Build history of the part. All positions in model axes, mm. Coordinates: 2 decimals unless noted, no trailing zeros. Write each loop counter-clockwise with the first axis right and the second up, starting at its lowest first coordinate (ties: lowest second). Pieces come first, ordered by that corner, then holes.
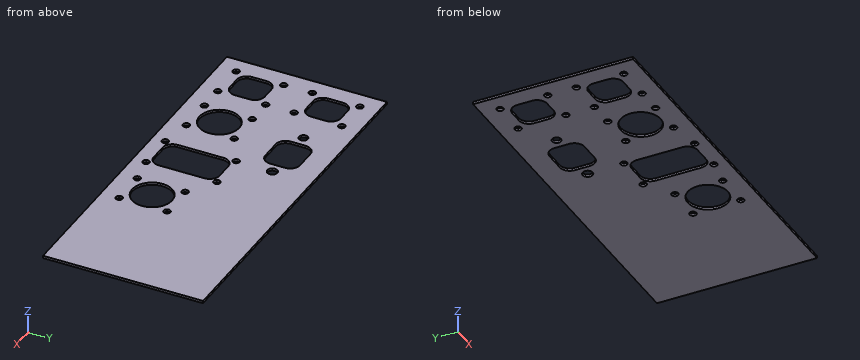
Autodesk Inventor part; units mm, degrees
ref_plane "YZ Plane" through (0, 0, 0) normal (1, 0, 0) x (0, 1, 0)
ref_plane "XZ Plane" through (0, 0, 0) normal (0, 1, 0) x (-1, 0, 0)
ref_plane "XY Plane" through (0, 0, 0) normal (0, 0, 1) x (1, 0, 0)
sketch "Sketch1" plane through (0, 0, 0) normal (0, 0, 1) x (1, 0, 0)
  line L0 (0, 0) -> (228.6, 0)
  line L1 (228.6, 0) -> (228.6, -101.6)
  line L2 (228.6, -101.6) -> (0, -101.6)
  line L3 (0, -101.6) -> (0, 0)
  dimension "d0" = 101.6
  dimension "d1" = 228.6
extrude "Extrusion1" add sketch "Sketch1" along normal blind 1.5875
sketch "Sketch2" plane through (0, 0, 1.5875) normal (0, 0, 1) x (1, 0, 0)
  line L0 (18.3388, -37.6555) -> (26.6192, -37.6555)
  line L1 (32.9692, -31.3055) -> (32.9692, -21.9075)
  line L2 (26.6192, -15.5575) -> (18.3388, -15.5575)
  line L3 (11.9888, -21.9075) -> (11.9888, -31.3055)
  arc A0 (11.9888, -31.3055) -> (18.3388, -37.6555) centre (18.3388, -31.3055) ccw
  arc A1 (18.3388, -15.5575) -> (11.9888, -21.9075) centre (18.3388, -21.9075) ccw
  arc A2 (32.9692, -21.9075) -> (26.6192, -15.5575) centre (26.6192, -21.9075) ccw
  arc A3 (26.6192, -37.6555) -> (32.9692, -31.3055) centre (26.6192, -31.3055) ccw
  circle A4 centre (10.9982, -41.783) radius 2.1463
  circle A5 centre (33.7058, -11.43) radius 2.1463
  circle A6 centre (33.7058, -41.783) radius 2.1463
  circle A7 centre (11.2522, -11.43) radius 2.1463
  line L4 (6.35, -46.863) -> (38.1, -46.863)
  line L5 (38.1, -46.863) -> (38.1, -6.35)
  line L6 (38.1, -6.35) -> (6.35, -6.35)
  line L7 (6.35, -6.35) -> (6.35, -46.863)
  line L8 (228.6, 0) -> (0, 0)
  line L9 (0, 0) -> (0, -101.6)
  point P0 (32.9692, -15.5575)
  point P1 (32.9692, -37.6555)
  point P2 (11.9888, -15.5575)
  dimension "d4" = 20.9804
  dimension "d5" = 22.098
  dimension "d6" = 6.35
  dimension "d7" = 4.2926
  dimension "d8" = 4.2926
  dimension "d9" = 4.2926
  dimension "d10" = 4.2926
  dimension "d11" = 0.9906
  dimension "d12" = 0.7366
  dimension "d13" = 0.7366
  dimension "d14" = 0.7366
  dimension "d15" = 4.1275
  dimension "d16" = 4.1275
  dimension "d17" = 4.1275
  dimension "d18" = 4.1275
  dimension "d19" = 31.75
  dimension "d20" = 40.513
  dimension "d21" = 5.08
  dimension "d22" = 4.6482
  dimension "d26" = 6.35
  dimension "d27" = 6.35
extrude "J9" cut sketch "Sketch2" against normal blind 1.5875 contours A0 L3 A1 L2 A2 L1 A3 L0 | A4 | A5 | A6 | A7
sketch "Sketch3" plane through (0, 0, 1.5875) normal (0, 0, 1) x (1, 0, 0)
  line L0 (67.183, -36.3982) -> (79.9084, -36.3982)
  line L1 (86.2584, -30.0482) -> (86.2584, -20.6502)
  line L2 (79.9084, -14.3002) -> (67.183, -14.3002)
  line L3 (60.833, -20.6502) -> (60.833, -30.0482)
  arc A0 (60.833, -30.0482) -> (67.183, -36.3982) centre (67.183, -30.0482) ccw
  arc A1 (79.9084, -36.3982) -> (86.2584, -30.0482) centre (79.9084, -30.0482) ccw
  arc A2 (86.2584, -20.6502) -> (79.9084, -14.3002) centre (79.9084, -20.6502) ccw
  arc A3 (67.183, -14.3002) -> (60.833, -20.6502) centre (67.183, -20.6502) ccw
  circle A4 centre (54.2417, -25.3492) radius 2.8067
  circle A5 centre (92.8497, -25.3492) radius 3.175
  line L4 (45.6692, -40.8432) -> (100.4062, -40.8432)
  line L5 (100.4062, -40.8432) -> (100.4062, -9.8552)
  line L6 (100.4062, -9.8552) -> (45.6692, -9.8552)
  line L7 (45.6692, -9.8552) -> (45.6692, -40.8432)
  line L8 (228.6, 0) -> (0, 0)
  line L9 (32.9692, -21.9075) -> (32.9692, -31.3055)
  dimension "d30" = 6.35
  dimension "d31" = 25.4254
  dimension "d32" = 22.098
  dimension "d33" = 5.6134
  dimension "d34" = 6.35
  dimension "d35" = 6.5913
  dimension "d36" = 6.5913
  dimension "d37" = 11.049
  dimension "d38" = 11.049
  dimension "d39" = 54.737
  dimension "d40" = 30.988
  dimension "d41" = 15.494
  dimension "d42" = 14.1478
  dimension "d98" = 12.7
  dimension "d99" = 9.8552
extrude "J8" cut sketch "Sketch3" against normal blind 1.5875 contours A0 L3 A3 L2 A2 L1 A1 L0 | A4 | A5
sketch "Sketch4" plane through (0, 0, 1.5875) normal (0, 0, 1) x (1, 0, 0)
  circle A0 centre (61.5442, -74.9935) radius 12.7
  circle A1 centre (50.3174, -90.17) radius 2.159
  circle A2 centre (50.3174, -59.817) radius 2.159
  circle A3 centre (72.771, -90.17) radius 2.159
  circle A4 centre (72.771, -59.817) radius 2.159
  line L0 (45.6692, -95.25) -> (77.4192, -95.25)
  line L1 (77.4192, -95.25) -> (77.4192, -54.737)
  line L2 (77.4192, -54.737) -> (45.6692, -54.737)
  line L3 (45.6692, -54.737) -> (45.6692, -95.25)
  line L4 (228.6, 0) -> (0, 0)
  line L5 (0, 0) -> (0, -101.6)
  line L6 (0, -101.6) -> (228.6, -101.6)
  line L7 (32.9692, -21.9075) -> (32.9692, -31.3055)
  dimension "d49" = 25.4
  dimension "d50" = 4.318
  dimension "d51" = 4.318
  dimension "d52" = 4.318
  dimension "d53" = 4.318
  dimension "d54" = 11.2268
  dimension "d55" = 11.2268
  dimension "d56" = 11.2268
  dimension "d57" = 11.2268
  dimension "d58" = 15.1765
  dimension "d59" = 15.1765
  dimension "d60" = 15.1765
  dimension "d61" = 15.1765
  dimension "d62" = 31.75
  dimension "d63" = 40.513
  dimension "d64" = 5.08
  dimension "d65" = 4.6482
  dimension "d69" = 6.35
  dimension "d97" = 12.7
extrude "J7" cut sketch "Sketch4" against normal blind 1.5875 contours A0 | A1 | A2 | A3 | A4
sketch "Sketch5" plane through (0, 0, 1.5875) normal (0, 0, 1) x (1, 0, 0)
  arc A0 (18.3388, -63.9445) -> (11.9888, -70.2945) centre (18.3388, -70.2945) ccw
  line L0 (32.9692, -79.6925) -> (32.9692, -70.2945)
  circle A1 centre (11.2522, -59.817) radius 2.1463
  line L1 (38.1, -54.737) -> (6.35, -54.737)
  line L2 (11.9888, -70.2945) -> (11.9888, -79.6925)
  line L3 (18.3388, -86.0425) -> (26.6192, -86.0425)
  line L4 (38.1, -95.25) -> (38.1, -54.737)
  line L5 (6.35, -54.737) -> (6.35, -95.25)
  line L6 (26.6192, -63.9445) -> (18.3388, -63.9445)
  circle A2 centre (33.7058, -59.817) radius 2.1463
  arc A3 (11.9888, -79.6925) -> (18.3388, -86.0425) centre (18.3388, -79.6925) ccw
  arc A4 (26.6192, -86.0425) -> (32.9692, -79.6925) centre (26.6192, -79.6925) ccw
  circle A5 centre (10.9982, -90.17) radius 2.1463
  circle A6 centre (33.7058, -90.17) radius 2.1463
  line L7 (6.35, -95.25) -> (38.1, -95.25)
  arc A7 (32.9692, -70.2945) -> (26.6192, -63.9445) centre (26.6192, -70.2945) ccw
  line L8 (228.6, 0) -> (0, 0)
  line L9 (0, 0) -> (0, -101.6)
  line L10 (0, -101.6) -> (228.6, -101.6)
  point P0 (11.9888, -63.9445)
  point P1 (32.9692, -63.9445)
  point P2 (32.9692, -86.0425)
  dimension "d72" = 20.9804
  dimension "d73" = 22.098
  dimension "d74" = 6.35
  dimension "d75" = 4.2926
  dimension "d76" = 4.2926
  dimension "d77" = 4.2926
  dimension "d78" = 4.2926
  dimension "d79" = 0.9906
  dimension "d80" = 0.7366
  dimension "d81" = 0.7366
  dimension "d82" = 0.7366
  dimension "d83" = 4.1275
  dimension "d84" = 4.1275
  dimension "d85" = 4.1275
  dimension "d86" = 4.1275
  dimension "d87" = 31.75
  dimension "d88" = 40.513
  dimension "d89" = 5.08
  dimension "d90" = 4.6482
  dimension "d93" = 6.35
  dimension "d94" = 6.35
extrude "J6" cut sketch "Sketch5" against normal blind 1.5875 contours L6 A7 L0 A4 L3 A3 L2 A0 | A1 | A2 | A5 | A6
sketch "Sketch6" plane through (0, 0, 1.5875) normal (0, 0, 1) x (1, 0, 0)
  line L0 (99.314, -49.9491) -> (110.1344, -49.9491)
  line L1 (116.4844, -56.2991) -> (116.4844, -85.4329)
  line L2 (110.1344, -91.7829) -> (99.314, -91.7829)
  line L3 (92.964, -85.4329) -> (92.964, -56.2991)
  arc A0 (92.964, -85.4329) -> (99.314, -91.7829) centre (99.314, -85.4329) ccw
  arc A1 (110.1344, -91.7829) -> (116.4844, -85.4329) centre (110.1344, -85.4329) ccw
  arc A2 (116.4844, -56.2991) -> (110.1344, -49.9491) centre (110.1344, -56.2991) ccw
  arc A3 (99.314, -49.9491) -> (92.964, -56.2991) centre (99.314, -56.2991) ccw
  circle A4 centre (92.7862, -48.387) radius 2.1463
  circle A5 centre (116.6622, -48.387) radius 2.1463
  circle A6 centre (116.6622, -93.345) radius 2.1463
  circle A7 centre (92.7862, -93.345) radius 2.1463
  line L4 (86.9442, -98.425) -> (122.5042, -98.425)
  line L5 (122.5042, -98.425) -> (122.5042, -43.307)
  line L6 (122.5042, -43.307) -> (86.9442, -43.307)
  line L7 (86.9442, -43.307) -> (86.9442, -98.425)
  line L8 (228.6, 0) -> (0, 0)
  line L9 (0, -101.6) -> (228.6, -101.6)
  circle A8 centre (61.5442, -74.9935) radius 12.7
  point P0 (92.964, -49.9491)
  point P1 (116.4844, -91.7829)
  point P2 (92.964, -91.7829)
  dimension "d100" = 23.5204
  dimension "d101" = 41.8338
  dimension "d102" = 6.35
  dimension "d103" = 0.1778
  dimension "d104" = 23.876
  dimension "d105" = 0.1778
  dimension "d106" = 1.5621
  dimension "d107" = 23.876
  dimension "d108" = 1.5621
  dimension "d109" = 1.5621
  dimension "d110" = 1.5621
  dimension "d111" = 35.56
  dimension "d112" = 55.118
  dimension "d113" = 5.08
  dimension "d114" = 5.842
  dimension "d115" = 4.2926
  dimension "d116" = 4.2926
  dimension "d117" = 4.2926
  dimension "d118" = 4.2926
  dimension "d121" = 3.175
  dimension "d122" = 12.7
extrude "J11" cut sketch "Sketch6" against normal blind 1.5875 contours L0 A2 L1 A1 L2 A0 L3 A3 | A4 | A5 | A6 | A7
sketch "Sketch7" plane through (0, 0, 1.5875) normal (0, 0, 1) x (1, 0, 0)
  circle A0 centre (156.2862, -90.17) radius 2.159
  line L0 (160.9344, -95.25) -> (160.9344, -54.737)
  circle A1 centre (145.0594, -74.9935) radius 12.7
  circle A2 centre (133.8326, -59.817) radius 2.159
  line L1 (160.9344, -54.737) -> (129.1844, -54.737)
  line L2 (129.1844, -95.25) -> (160.9344, -95.25)
  circle A3 centre (156.2862, -59.817) radius 2.159
  circle A4 centre (133.8326, -90.17) radius 2.159
  line L3 (129.1844, -54.737) -> (129.1844, -95.25)
  line L4 (116.4844, -56.2991) -> (116.4844, -85.4329)
  line L5 (0, -101.6) -> (228.6, -101.6)
  point P0 (0, 0)
  dimension "d125" = 25.4
  dimension "d126" = 4.318
  dimension "d127" = 4.318
  dimension "d128" = 4.318
  dimension "d129" = 4.318
  dimension "d130" = 11.2268
  dimension "d131" = 11.2268
  dimension "d132" = 11.2268
  dimension "d133" = 11.2268
  dimension "d134" = 15.1765
  dimension "d135" = 15.1765
  dimension "d136" = 15.1765
  dimension "d137" = 15.1765
  dimension "d138" = 31.75
  dimension "d139" = 40.513
  dimension "d140" = 5.08
  dimension "d141" = 4.6482
  dimension "d144" = 12.7
  dimension "d146" = 6.35
extrude "J4" cut sketch "Sketch7" against normal blind 1.5875 contours A0 | A1 | A2 | A3 | A4
equation "\"d27\" = d26"
equation "\"d37\" = 0.5 * d32"
equation "\"d41\" = 0.5 * d40"
equation "\"d94\" = d93"
properties part number "Plug-in Plate"
1. Saw through at A-A on y = -11.43. List the corners of the cut face in (x, z), plus the area to 3 significant figures.
Computed values:
outline: (0, 0) - (9.11, 0) - (9.11, 1.59) - (0, 1.59) - close; (13.4, 0) - (31.56, 0) - (31.56, 1.59) - (13.4, 1.59) - close; (35.85, 0) - (228.6, 0) - (228.6, 1.59) - (35.85, 1.59) - close
area: 349 mm2
2. Saw through at B-B on z = 0.25. State how many separate pieces and enclosed holes the cut face has, plus the area to 3 significant figures.
Computed values:
separate pieces: 1
enclosed holes: 28
area: 19,500 mm2
3. Probe line 1 along X through (y, z) = (-75.5, 0.3); line 2 along X through (y, z) = (-48.5, 1.5); line 3 along X through (y, z) = (-20.5, 0.1). List the from-to ranges inside material, lowest first.
Computed values:
line 1: x = 0 to 11.99, 32.97 to 48.85, 74.23 to 92.96, 116.48 to 132.37, 157.75 to 228.6
line 2: x = 0 to 90.64, 94.93 to 114.52, 118.81 to 228.6
line 3: x = 0 to 12.15, 32.81 to 60.83, 86.26 to 228.6
4. Flat gauge pin, fed straight in: pin 1 (2.5 mm diameter, centred on x = 11.25, y = -11.43, fed in from +Z). Where does the tip first touch, or does it go through?
Computed values:
pin 1: passes through
